```python
from build123d import *

# Parameters (mm, degrees)
SKETCH1_W           = 50
SKETCH1_H           = 85
BOSS_EXTRUDE1_DEPTH = 3
SKETCH4_W           = 3
SKETCH4_H           = 85
BOSS_EXTRUDE2_DEPTH = 50
CUT_EXTRUDE1_DEPTH  = 50
FILLET2_R           = 10
SKETCH6_R           = 5
CUT_EXTRUDE2_DEPTH  = 50
SKETCH7_R           = 2.5
CUT_EXTRUDE3_DEPTH  = 20


with BuildPart() as part:
    # Sketch1 → Boss-Extrude1 (new body)
    with BuildSketch(Plane.XY):
        Rectangle(SKETCH1_W, SKETCH1_H)
    extrude(amount=BOSS_EXTRUDE1_DEPTH)

    # Sketch4 → Boss-Extrude2 (add)
    with BuildSketch(Plane(origin=(0, 0, 0), x_dir=(-1, 0, 0), z_dir=(0, 0, -1))):
        with Locations((-23.5, 0)):
            Rectangle(SKETCH4_W, SKETCH4_H)
        with Locations((23.5, 0)):
            Rectangle(SKETCH4_W, SKETCH4_H)
    extrude(amount=BOSS_EXTRUDE2_DEPTH)

    # Sketch5 → Cut-Extrude1 (cut)
    with BuildSketch(Plane(origin=(25, 0, 0), x_dir=(0, 0, -1), z_dir=(1, 0, 0))):
        Polygon((50, 0), (-3, -42.5), (50, -42.5), align=None)
        Polygon((-3, 42.5), (50, 0), (50, 42.5), align=None)
    extrude(amount=-CUT_EXTRUDE1_DEPTH, mode=Mode.SUBTRACT)

    # Fillet2
    fillet2_edges = [part.edges().sort_by_distance(p)[0] for p in [
        (23.5, 0, -50),
        (-23.5, 0, -50),
    ]]
    fillet(fillet2_edges, radius=FILLET2_R)

    # Sketch6 → Cut-Extrude2 (cut)
    with BuildSketch(Plane(origin=(25, 0, 0), x_dir=(0, 0, -1), z_dir=(1, 0, 0))):
        with Locations(Location((36.614754057, 0, 0), (0, 0, 90))):
            Circle(SKETCH6_R)
    extrude(amount=-CUT_EXTRUDE2_DEPTH, mode=Mode.SUBTRACT)

    # Sketch7 → Cut-Extrude3 (cut)
    with BuildSketch(Plane.XY.offset(3)):
        with Locations((0, 15)):
            Circle(SKETCH7_R)
        with Locations((0, -15)):
            Circle(SKETCH7_R)
    extrude(amount=-CUT_EXTRUDE3_DEPTH, mode=Mode.SUBTRACT)


solid = part.part
```
Geometry: final body of the model. Coordinates: model frame, mm. A direction names the side the tool comes from. Give positions to 0.01 mm unless a question says otherwise; leave off trailing zeros. Loops run counter-clockwise (first coordinate to the right, second up) from the corner with the lowest first, then second, coordinate; pieces in that order, holes last. Notation, with made-up numbers: (41.5, 71.5) - (73.5, 71.5) arc R37 cw to (73.5, 109.5) - close; hole circle Ø7 at (41.25, 77.5). An arc over 180 degrees is marked (long way). Answer as CSV lines item,"result". Start each with the question number.
(1) Mould query, pull axis Z, two halves, no side actions, for faces 3 (the face through (-22, -1, -17)), 4 (the face through (-23.521, -0.125, -44.014)), 5 (the face through (-23.479, -0.651, -31.657)). Classes: +Z half, -Z half, draft (parallel to the pull), parting line (faces both ways), or undercut.
(2) Section query A-A (x = 0). Output: boundary loops of the cut face in (y, z).
(3) Section query C-C (z = -26). Output: boundary loops of the cut face in (x, y), and give its area (3 significant figures).
(4) Section query D-D (z = -35.5). Output: boundary loops of the cut face in (x, y).
(5) Ray query, line 1 along X through (y, z) = (-21.5, -14.5); line 2 along Y through (x, z) = (0, 1.6); line 3 along Y through (x, z) = (0, 2.05). Return the intervals inside material, ascending. Write a range as [from, to].
(6) Section query B-B (y = 15). Output: boundary loops of the cut face in (x, z), and give its area (3 significant figures).
(7) Pin query (flat end, axial travel): P1, Ø4.5, axis at x = 0, y = -15, coming from the +Z side; P2, Ø4, axis at x = 0.5, y = 29.5, coming from the -Z side. Return the tip coordinate at first contact, or that it passes through.
(8) Reachability of faces 1 (the face through (23.479, -0.125, -44.014)), 2 (the face through (22, -1, -17)) from +Z, -Z, +X, -X, +Y, -Y: full face, straight path, thin tool, end or side. Return the list, or none.
Worked answers:
1,face 3,"draft"
1,face 4,"-Z half"
1,face 5,"undercut"
2,outline,"(-42.5, 3) - (-40.09, 0) - (-17.5, 0) - (-17.5, 3) - close; (-12.5, 0) - (12.5, 0) - (12.5, 3) - (-12.5, 3) - close; (17.5, 0) - (40.09, 0) - (42.5, 3) - (17.5, 3) - close"
3,outline,"(-25, -19.25) - (-22, -19.25) - (-22, 19.25) - (-25, 19.25) - close; (22, -19.25) - (25, -19.25) - (25, 19.25) - (22, 19.25) - close"
3,area,"231 mm^2"
4,outline,"(-25, -11.63) - (-22, -11.63) - (-22, -4.87) - (-25, -4.87) - close; (-25, 4.87) - (-22, 4.87) - (-22, 11.63) - (-25, 11.63) - close; (22, -11.63) - (25, -11.63) - (25, -4.87) - (22, -4.87) - close; (22, 4.87) - (25, 4.87) - (25, 11.63) - (22, 11.63) - close"
5,line 1,"x = [-25, -22], [22, 25]"
5,line 2,"y = [-41.38, -17.5], [-12.5, 12.5], [17.5, 41.38]"
5,line 3,"y = [-41.74, -17.5], [-12.5, 12.5], [17.5, 41.74]"
6,outline,"(-25, -31.29) - (-22, -31.29) - (-22, 0) - (-2.5, 0) - (-2.5, 3) - (-25, 3) - close; (2.5, 0) - (22, 0) - (22, -31.29) - (25, -31.29) - (25, 3) - (2.5, 3) - close"
6,area,"323 mm^2"
7,P1,"passes through"
7,P2,"stops at z = 0"
8,face 1,"-Z, +X, -X"
8,face 2,"-Z, +Y, -Y"
